The model under review builds one solid part; all positions refer to its coordinate system, in mm. A direction names the side the tool comes from. Give positions to 0.01 mm unless a question says otherwise; leave off trailing zeros. Loops run counter-clockwise (first coordinate to the right, second up) from the corner with the lowest first, then second, coordinate; pieces in that order, holes last. Notation, with made-up numbers: M 32.25,-0.75 L 62.25,-0.75 A14 cw 62.25,23.25 Z; hole C -28,13.5 d4. An arc over 180 degrees is marked long. One line per item, written item: value. Start each with the question number.
Q1. We need section C-C on y = -114.5. Write out the cut boundary in (x, z) (1 decimal), plus the area to 3 significant figures.
Q2. Mouldability with a two-part tool opening along Z and no side actions: class faces 4 (the face through (-11, -101.6, 0)), 5 (the face through (-11, -6.35, -7)), 6 (the face through (-3.441, -3.131, -15.497)) as released by +Z, released by -Z, zero draft, split by the parting line, or undercut.
Q3. For faces 1 (the face through (0, -152.4, 0)), 2 (the face through (12.05, -78.35, 3.8)), 3 (the face through (-11, -127, -3.175)), list the 3-axis set-ups (+Z, -Z, +X, -X, +Y, -Y) from which the entire face can be reached by the end or side of a thin tool; tool diameter is ignored.
Q4. We need section D-D on z = -9. Write out the cut boundary in (x, y), plus the area to 3 significant figures.
Q5. To check wall thickness, follow line 1 along Z through (x, y) = (0, -67); line 2 along Y through (x, z) = (8.5, -13); line 3 along Z through (x, y) = (-9.5, -107) (3 decimals). State the ranges of each line that lie inside material, in increasing order. Write a range as from..to.
Q6. For pin 1 (12 mm diameter, centred on y = -38, z = 1.5, fed in from -X); pin 2 (1.5 mm diameter, centred on x = 9, y = -19.5, fed in from -Z); pin 3 (0.8 mm diameter, centred on x = -11, y = -114.5, fed in from +Z), all flat-tipped, find the tip position at first contact; note any pin that passes through.
```python
from build123d import *

# Parameters (mm, degrees)
F0_R     = 15.875
F0_R_2   = 12.6365
F1_DEPTH = 6.35
F2_R     = 12.6365
F3_DEPTH = 152.4
F5_DEPTH = 50.8


with BuildPart() as f1:
    # F0 (on Front) → F1 (new body)
    with BuildSketch(Plane.XZ):
        Circle(F0_R)
        Circle(F0_R_2, mode=Mode.SUBTRACT)
    extrude(amount=F1_DEPTH)

    # F2 (on Front) → F3 (join)
    with BuildSketch(Plane.XZ):
        Circle(F2_R)
    extrude(amount=F3_DEPTH)

    # F4 (on face) → F5 (cut)
    with BuildSketch(Plane.XZ.offset(152.4)):
        with BuildLine():
            Line((-9.4615, 3.175), (-12.2311286172, 3.175))
            ThreePointArc((-12.2311286172, 3.175), (-12.5347474849, 1.6003867469), (-12.6365, 0))
            ThreePointArc((-12.6365, 0), (-12.5347474849, -1.6003867469), (-12.2311286172, -3.175))
            Line((-12.2311286172, -3.175), (-9.4615, -3.175))
            Line((-9.4615, -3.175), (-9.4615, 3.175))
        make_face()
    extrude(amount=-F5_DEPTH, mode=Mode.SUBTRACT)


solid = f1.part
```
Solved:
1. outline: M -12.2,-3.2 A12.6 ccw long -12.2,3.2 L -9.5,3.2 L -9.5,-3.2 Z
1. area: 482 mm2
2. face 4: undercut
2. face 5: zero draft
2. face 6: split by the parting line
3. face 1: +Z, -Z, +X, -X, -Y
3. face 2: -Y
3. face 3: -X, -Y
4. outline: M -13.08,-6.35 L -8.87,-6.35 L -8.87,-152.4 L 8.87,-152.4 L 8.87,-6.35 L 13.08,-6.35 L 13.08,0 L -13.08,0 Z
4. area: 2,760 mm2
5. line 1: -12.64..12.64
5. line 2: -6.35..0
5. line 3: -8.333..-3.175, 3.175..8.333
6. pin 1: x = -12.64
6. pin 2: z = -9.57
6. pin 3: z = 6.88
